For this review, take the finished solid that the model builds, in its own axes (mm). A direction names the side the tool comes from. Give positions to 0.01 mm unless a question says otherwise; leave off trailing zeros. Order: outer loops, then holes, each group sorted by start corner. A loop starts at its lowest first (then second) coordinate and runs counter-clockwise, first axis right, second up. Notation, with made-up numbers: (63, 69) - (102, 69) arc R29 ccw to (102, 105) - close; hole circle Ø2 at (71, 38.5). An arc over 180 degrees is marked (long way). Use a Markdown table: item, result. Add a question column.
1) We need section C-C on x = 117.5. Write out the cut boundary in (y, z), then the cut area to 3 significant figures.
2) Mouldability with a two-part tool opening along Y and no side actions: class faces 1 (the face through (0, -1, 1)), 2 (the face through (138, 70, -1)), 3 (the face through (138, 35, -10)) as released by +Y, released by -Y, zero draft, split by the parting line, or undercut.
3) We need section A-A on z = 18. Write out the cut boundary in (x, y), then the cut area to 3 significant figures.
4) Wall thickness on L1, parallel to Z at x = 48, y = 25.5: over which ranges is the line inside the solid? List them lowest first.
5) Machinability: for faces 4 (the face through (138, -1, 70)), 5 (the face through (138, 60, -35)), which of the approach directions +Z, -Z, +X, -X, +Y, -Y give a long, thin tool a straight path to every point of the face, cutting with its end or side? Answer none if there is none.
```python
from build123d import *

# Parameters (mm, degrees)
SKETCH_W   = 140
SKETCH_H   = 140
SKETCH_W_2 = 50
SKETCH_H_2 = 50
PAD_DEPTH  = 280


with BuildPart() as part:
    # Sketch → Pad (new body)
    with BuildSketch(Plane.YZ):
        Rectangle(SKETCH_W, SKETCH_H)
        with Locations((35, 35)):
            Rectangle(SKETCH_W_2, SKETCH_H_2, mode=Mode.SUBTRACT)
        with Locations((-35, 35)):
            Rectangle(SKETCH_W_2, SKETCH_H_2, mode=Mode.SUBTRACT)
        with Locations((-35, -35)):
            Rectangle(SKETCH_W_2, SKETCH_H_2, mode=Mode.SUBTRACT)
        with Locations((35, -35)):
            Rectangle(SKETCH_W_2, SKETCH_H_2, mode=Mode.SUBTRACT)
    extrude(amount=PAD_DEPTH)


solid = part.part
```
Checked values:
| question | item | result |
|---|---|---|
| 1 | outline | (-70, -70) - (70, -70) - (70, 70) - (-70, 70) - close; hole (-60, -60) - (-10, -60) - (-10, -10) - (-60, -10) - close; hole (-60, 10) - (-10, 10) - (-10, 60) - (-60, 60) - close; hole (10, -60) - (60, -60) - (60, -10) - (10, -10) - close; hole (10, 10) - (60, 10) - (60, 60) - (10, 60) - close |
| 1 | area | 9,600 mm² |
| 2 | face 1 | zero draft |
| 2 | face 2 | released by +Y |
| 2 | face 3 | undercut |
| 3 | outline | (0, -70) - (280, -70) - (280, -60) - (0, -60) - close; (0, -10) - (280, -10) - (280, 10) - (0, 10) - close; (0, 60) - (280, 60) - (280, 70) - (0, 70) - close |
| 3 | area | 11,200 mm² |
| 4 | L1 | -70 to -60, -10 to 10, 60 to 70 |
| 5 | face 4 | +Z, +X, -X, +Y, -Y |
| 5 | face 5 | +X, -X |
